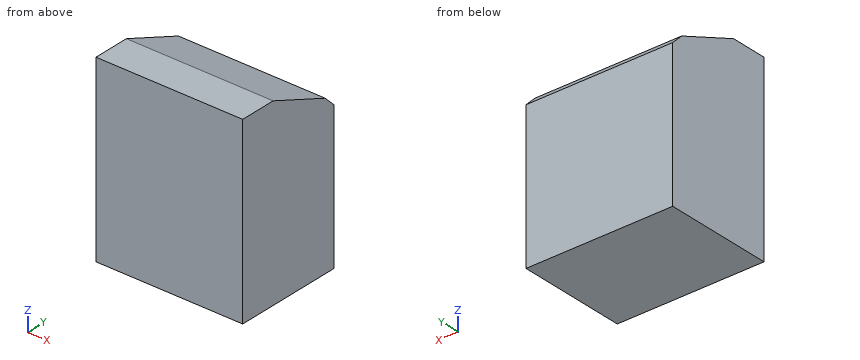
```python
from build123d import *

# Parameters (mm, degrees)
F0_W     = 20.1190489383
F0_H     = 15
F1_DEPTH = 25
F2_SIZE  = 5
F3_SIZE  = 5


with BuildPart() as f1:
    # F0 (on Top) → F1 (new body)
    with BuildSketch(Plane.XY):
        with Locations((-10.0595244691, 3.5714283609)):
            Rectangle(F0_W, F0_H)
    extrude(amount=F1_DEPTH)

    # F2
    f2_edges = [f1.edges().sort_by_distance(p)[0] for p in [
        (-10.059524, 11.071428, 25),
    ]]
    chamfer(f2_edges, length=F2_SIZE)

    # F3
    f3_edges = [f1.edges().sort_by_distance(p)[0] for p in [
        (-10.059524, 6.071428, 25),
    ]]
    chamfer(f3_edges, length=F3_SIZE)


solid = f1.part
```
The listing builds one solid part. Answer for the finished solid, in the listing's coordinates (mm). Coordinates: 2 decimals unless noted, no trailing zeros. Write each loop counter-clockwise with the first axis right and the second up, starting at its lowest first coordinate (ties: lowest second). Pieces come first, ordered by that corner, then holes. Notation, with made-up numbers: M -36,56.25 L 23,56.25 A26 cw 23,85.25 Z; hole C 78,2 d7. An arc over 180 degrees is marked long. Use a Markdown table: item, result. Add a question column.
1. Section B-B (z = 22.75) is taken. Give the vertices of the cut face in (x, y).
2. Section A-A (x = -18) is taken. Give the vertices of the cut face in (y, z), plus the area to 3 significant figures.
3. Section C-C (y = 7.25) is taken. Give the vertices of the cut face in (x, z).
4. Straight lines are drawn through the part: line 1 along Z through (x, y) = (-15.5, 8.5); line 2 along Z through (x, y) = (-10.5, 6.75); line 3 along Y through (x, z) = (-5.75, 20.75). For each, find the intervals that lie inside material, in ascending order. Write a range as [from, to].
Data:
| question | item | result |
|---|---|---|
| 1 | outline | M -20.12,-3.93 L 0,-3.93 L 0,6.5 L -20.12,6.5 Z |
| 2 | outline | M -3.93,0 L 11.07,0 L 11.07,20 L 9.61,21.46 L 1.07,25 L -3.93,25 Z |
| 2 | area | 354 mm2 |
| 3 | outline | M -20.12,0 L 0,0 L 0,22.44 L -20.12,22.44 Z |
| 4 | line 1 | z = [0, 21.92] |
| 4 | line 2 | z = [0, 22.65] |
| 4 | line 3 | y = [-3.93, 10.32] |
